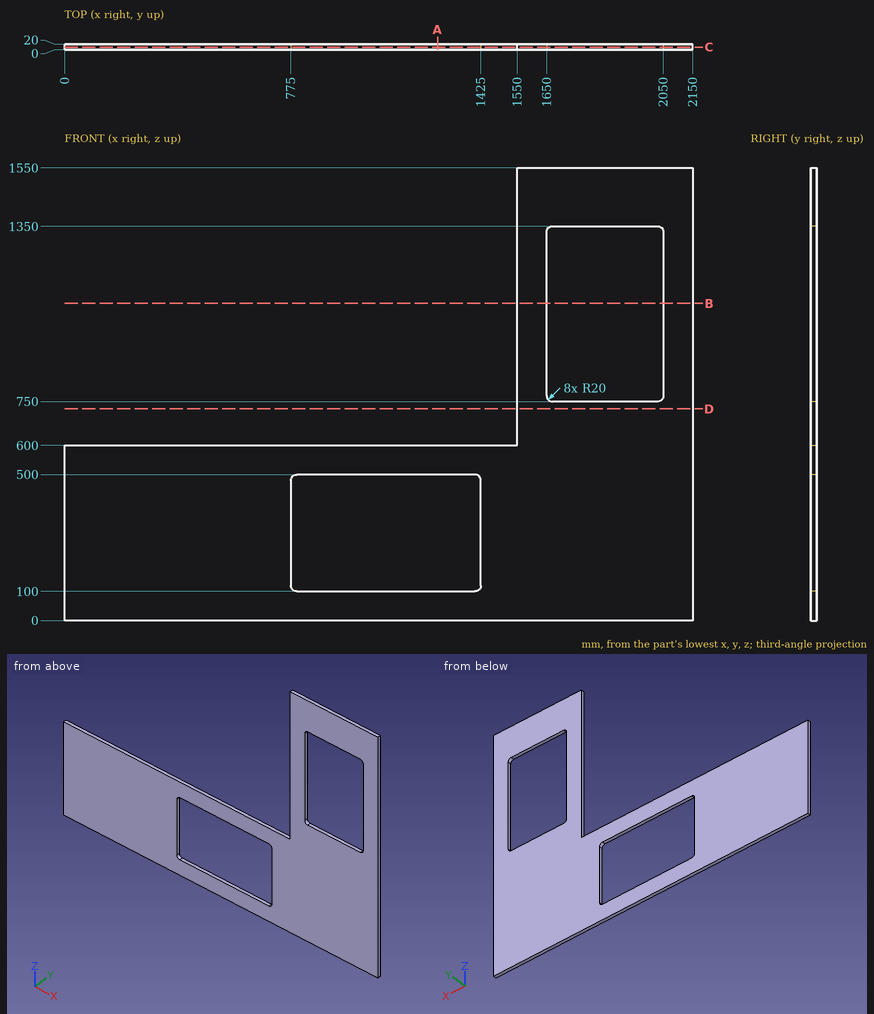
Verification items for this drawing (mm, ordinates from the low corner). Give positions to 0.01 mm unless a question says otherwise; leave off trailing zeros. Write each loop counter-clockwise with the first axis right and the second up, starting at its lowest first coordinate (ties: lowest second). Pieces come first, ordered by that corner, then holes.
1) Section check B-B, the plane z = 1086.5. Record the boundary of the cut face in (x, y), and give its area (3 significant figures).
2) Material ranges on L1, parallel to Z at x = 1753.5, y = 1.75; L2, parallel to Z at x = 1203, y = 8.25; L3, parallel to X at y = 14.75, z = 1124, recorded low to high.
3) Section check D-D, the plane z = 725. Record the boundary of the cut face in (x, y).
4) Section check A-A, the plane x = 1277.5. Record the boundary of the cut face in (y, z), and give its area (3 significant figures).
5) Section check C-C, the plane y = 9. Record the boundary of the cut face in (x, z), and give its area (3 significant figures).
6) Gauge pin test, flat ends, axial feed: pin 1 (8 mm diameter, centred on x = 1419, y = 16, fed in from +Z); pin 2 (5 mm diameter, centred on y = 6, z = 1259.5, fed in from -X). Record the tip position at first contact, or that the pin passes through.
Computed:
1. outline: (1550, 0) - (1650, 0) - (1650, 20) - (1550, 20) - close; (2050, 0) - (2150, 0) - (2150, 20) - (2050, 20) - close
1. area: 4,000 mm2
2. L1: z = 0 to 750, 1350 to 1550
2. L2: z = 0 to 100, 500 to 600
2. L3: x = 1550 to 1650, 2050 to 2150
3. outline: (1550, 0) - (2150, 0) - (2150, 20) - (1550, 20) - close
4. outline: (0, 0) - (20, 0) - (20, 100) - (0, 100) - close; (0, 500) - (20, 500) - (20, 600) - (0, 600) - close
4. area: 4,000 mm2
5. outline: (0, 0) - (2150, 0) - (2150, 1550) - (1550, 1550) - (1550, 600) - (0, 600) - close; hole (775, 120) arc R20 ccw to (795, 100) - (1405, 100) arc R20 ccw to (1425, 120) - (1425, 480) arc R20 ccw to (1405, 500) - (795, 500) arc R20 ccw to (775, 480) - close; hole (1650, 770) arc R20 ccw to (1670, 750) - (2030, 750) arc R20 ccw to (2050, 770) - (2050, 1330) arc R20 ccw to (2030, 1350) - (1670, 1350) arc R20 ccw to (1650, 1330) - close
5. area: 1,360,000 mm2
6. pin 1: stops at z = 600
6. pin 2: stops at x = 1550
